Autodesk Inventor part; units mm, degrees
ref_plane "YZ Plane" through (0, 0, 0) normal (1, 0, 0) x (0, 1, 0)
ref_plane "XZ Plane" through (0, 0, 0) normal (0, 1, 0) x (-1, 0, 0)
ref_plane "XY Plane" through (0, 0, 0) normal (0, 0, 1) x (1, 0, 0)
sketch "Sketch1" plane through (0, 0, 0) normal (0, 0, 1) x (1, 0, 0)
  line L0 (0, 0) -> (0, 15)
  line L1 (0, 15) -> (2, 15)
  line L2 (2, 15) -> (2, 13)
  line L3 (2, 13) -> (10, 13)
  line L4 (10, 13) -> (10, 0)
  line L5 (10, 0) -> (0, 0)
  dimension "d0" = 2
  dimension "d1" = 8
  dimension "d2" = 30
  dimension "d3" = 26
revolve "Revolution1" add sketch "Sketch1" angle 360 about axis through (10, 0, 0) along (-1, 0, 0)
fillet "Fillet1" radius 1 1 edges at (0, -15, 0)
sketch "Sketch2" plane through (10, 0, 0) normal (1, 0, 0) x (0, 0, -1)
  circle A0 centre (0, 0) radius 13
  point P0 (0, 0)
hole "Hole1" at (10, 0, 0) direction (-1, 0, 0) diameter 20 depth 10
properties part number "101 part 3" material "Copper, Alloy"
For this review, take the finished solid that the model builds, in its own axes (mm). A direction names the side the tool comes from. Round coordinates to 2 decimals unless told otherwise and drop trailing zeros. Order: outer loops, then holes, each group sorted by start corner. A loop starts at its lowest first (then second) coordinate and runs counter-clockwise, first axis right, second up. Notation, with made-up numbers: (76, -12.75) -> (99, -12.75) arc R22 cw to (99, 6.25) -> close; hole circle Ø2 at (31, -2). An arc over 180 degrees is marked (long way). Write item = value, one per line. Start each with the question number.
1) Insertion check: pin 1 (2 mm diameter, centred on x = 5.5, y = -5, fed in from +Z); pin 2 (1.5 mm diameter, centred on x = 4.5, y = 6.5, fed in from +Z); pin 3 (1.5 mm diameter, centred on x = 7.5, y = -7, fed in from -Z). Each pin has a flat end and moves straight along its axis. Give the tip position at first contact, or say it passes through.
2) Take a section at C-C on x = 5.75. State the section outline as (y, z) points.
3) Tool access review of faces 1 (the face through (6.056, -10.316, -7.91)), 2 (the face through (0, -3, -10)): name each direction out of +Z, -Z, +X, -X, +Y, -Y from which nothing blocks a thin tool from reaching the whole face with its end or side.
4) Take a section at A-A on y = 0. State the section outline as (x, z) points, plus the area to 3 significant figures.
5) To check wall thickness, follow line 1 (Y direction, x = 4, z = 0); line 2 (X direction, y = 10.75, z = -7.5). State the ranges of each line that lie inside material, in increasing order. Write a range as from..to.
6) The part is to be moulded in two halves that separate along Z. For faces 3 (the face through (1.507, -14.985, 0.66)), 4 (the face through (4.93, 9.76, 2.17)), 5 (the face through (2, -0.1, -13.4)), say which applies: +Z half, -Z half, draft (parallel to the pull), parting line (faces both ways), or undercut.
Verdict:
q1.pin_1 = 12.37
q1.pin_2 = 11.66
q1.pin_3 = -11.4
q2.outline = circle Ø26 at (0, 0); hole circle Ø20 at (0, 0)
q3.face_1 = +X
q3.face_2 = +Z, -Z, -X, +Y, -Y
q4.outline = (0, -14) arc R1 ccw to (1, -15) -> (2, -15) -> (2, -13) -> (10, -13) -> (10, -10) -> (0, -10) -> close; (0, 10) -> (10, 10) -> (10, 13) -> (2, 13) -> (2, 15) -> (1, 15) arc R1 ccw to (0, 14) -> close
q4.area = 67.6 mm2
q5.line_1 = -13..-10, 10..13
q5.line_2 = 0..2
q6.face_3 = parting line
q6.face_4 = undercut
q6.face_5 = draft
